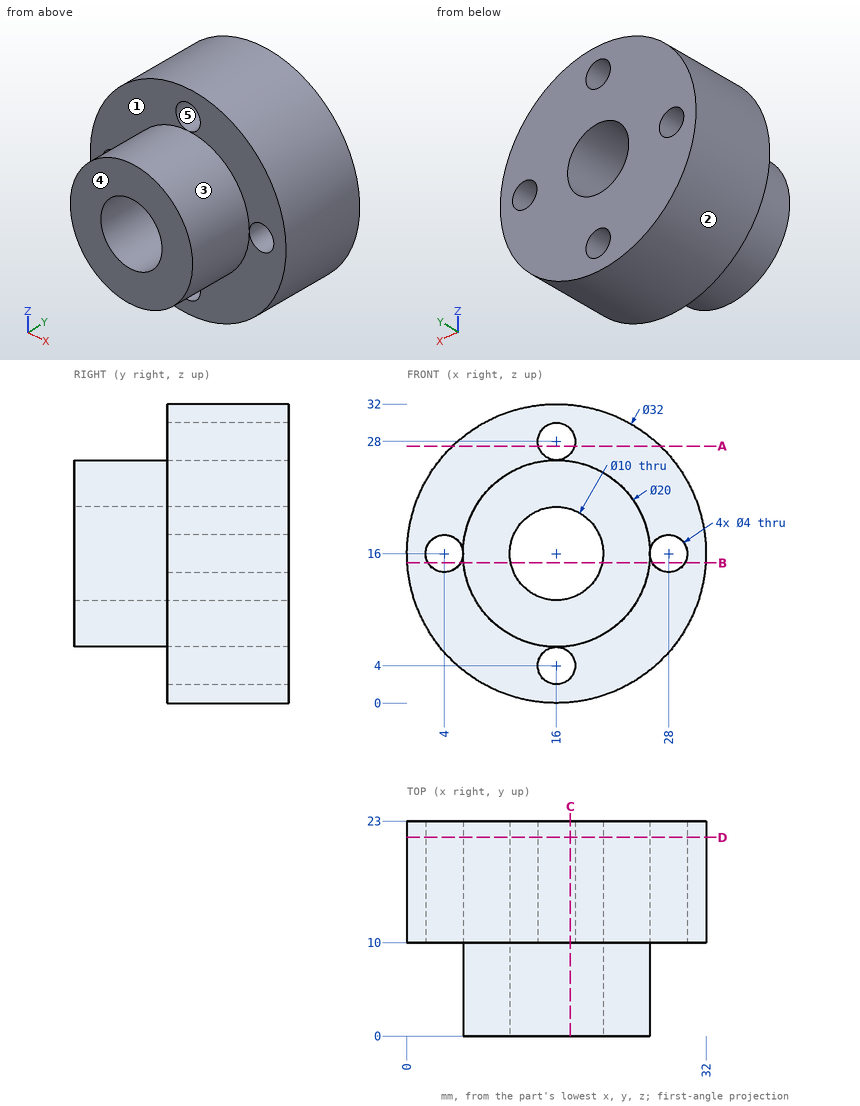
The drawing under review shows one solid part. Ordinate dimensions are in mm from its lowest x, y, z. A direction names the side the tool comes from. Round coordinates to 2 decimals unless told otherwise and drop trailing zeros. Loops run counter-clockwise (first coordinate to the right, second up) from the corner with the lowest first, then second, coordinate; pieces in that order, holes last. Notation, with made-up numbers: M 25,68 L 77,68 A32 cw 77,96 Z; hole C 75.25,-9 d6. An arc over 180 degrees is marked long. Answer as CSV lines item,"result". Start each with the question number.
Item 1: Mouldability with a two-part tool opening along X and no side actions: class the marked faces 3, 4 and 5 as released by +X, released by -X, zero draft, split by the parting line, or undercut.
Item 2: Wall thickness on line 1 (X direction, y = 13.5, z = 16); line 2 (Y direction, x = 18, z = 26); line 3 (X direction, y = 19.25, z = 20): over which ranges is each line inside the solid? List them lowest first. Write a range as [from, to].
Item 3: Consider section B-B (z = 15). Write out the cut boundary in (x, y), then the cut area to 3 significant figures.
Item 4: Consider section D-D (y = 21.25). Write out the cut boundary in (x, z).
Item 5: Consider section A-A (z = 27.5). Write out the cut boundary in (x, y).
Item 6: Consider section C-C (x = 17.5). Write out the cut boundary in (y, z), then the cut area to 3 significant figures.
Item 7: For the marked faces 1 and 2, list the 3-axis set-ups (+Z, -Z, +X, -X, +Y, -Y) from which the entire face can be reached by the end or side of a thin tool; tool diameter is ignored.
Item 8: Insertion check: P1, Ø10, axis at y = 4, z = 16, coming from the +X side; P2, Ø2, axis at y = 6.5, z = 6.5, coming from the +X side; P3, Ø10, axis at y = 6, z = 3.5, coming from the +X side; P4, Ø2.5, axis at x = 28, z = 16, coming from the -Y side. Each pin has a flat end and moves straight along its axis. Give the tip position at first contact, or say it passes through.
Answer:
1,face 3,"split by the parting line"
1,face 4,"zero draft"
1,face 5,"undercut"
2,line 1,"x = [0, 2], [6, 11], [21, 26], [30, 32]"
2,line 2,"y = [10, 23]"
2,line 3,"x = [0.51, 13], [19, 31.49]"
3,outline,"M 0.03,10 L 2.27,10 L 2.27,23 L 0.03,23 Z; M 5.73,10 L 6.05,10 L 6.05,0 L 11.1,0 L 11.1,23 L 5.73,23 Z; M 20.9,0 L 25.95,0 L 25.95,10 L 26.27,10 L 26.27,23 L 20.9,23 Z; M 29.73,10 L 31.97,10 L 31.97,23 L 29.73,23 Z"
3,area,"299 mm^2"
4,outline,"C 16,16 d32; hole C 4,16 d4; hole C 16,16 d10; hole C 16,4 d4; hole C 16,28 d4; hole C 28,16 d4"
5,outline,"M 4.88,10 L 14.06,10 L 14.06,23 L 4.88,23 Z; M 17.94,10 L 27.12,10 L 27.12,23 L 17.94,23 Z"
6,outline,"M 0,6.11 L 10,6.11 L 10,5.32 L 23,5.32 L 23,11.23 L 0,11.23 Z; M 0,20.77 L 23,20.77 L 23,26.68 L 10,26.68 L 10,25.89 L 0,25.89 Z; M 10,0.07 L 23,0.07 L 23,2.68 L 10,2.68 Z; M 10,29.32 L 23,29.32 L 23,31.93 L 10,31.93 Z"
6,area,"324 mm^2"
7,face 1,"-Y"
7,face 2,"+Y, -Y"
8,P1,"stops at x = 26"
8,P2,"stops at x = 21.27"
8,P3,"stops at x = 28.87"
8,P4,"passes through"
